from build123d import *

# Parameters (mm, degrees)
SKETCH_1_R               = 28.35
EXTRUDE_1_DEPTH          = 6
SKETCH_2_R               = 16
EXTRUDE_2_DEPTH          = 12
SKETCH_3_R               = 6.5
CUT_EXTRUDE_1_DEPTH      = 19
HOLE_WIZARD_M5_2_D       = 4.2
PATTERN_CIRCULAR_1_COUNT = 6
CUT_EXTRUDE_3_REACH      = 46.35
SKETCH_6_R               = 2.1


with BuildPart() as part:
    # Sketch 1 → Extrude 1 (new body)
    with BuildSketch(Plane.XY):
        Circle(SKETCH_1_R)
    extrude(amount=EXTRUDE_1_DEPTH)

    # Sketch 2 → Extrude 2 (add)
    with BuildSketch(Plane.XY.offset(6)):
        Circle(SKETCH_2_R)
    extrude(amount=EXTRUDE_2_DEPTH)

    # Sketch 3 → Cut-Extrude 1 (cut, through all)
    with BuildSketch(Plane.XY.offset(18)):
        Circle(SKETCH_3_R)
    extrude(amount=-CUT_EXTRUDE_1_DEPTH, mode=Mode.SUBTRACT)

    # Hole Wizard M5 _2 (through all)
    with Locations(Plane(origin=(0, 0, 0), x_dir=(-1, 0, 0), z_dir=(0, 0, -1))):
        with Locations((0, 23.75)):
            hole_wizard_m5_2 = Hole(HOLE_WIZARD_M5_2_D / 2)

    # Pattern Circular 1: Hole Wizard M5 _2 ×6 about axis
    pattern_circular_1_axis = Axis((0, 0, 0), (0, 0, 1))
    for i in range(1, PATTERN_CIRCULAR_1_COUNT):
        add(hole_wizard_m5_2.rotate(pattern_circular_1_axis, i * 360 / PATTERN_CIRCULAR_1_COUNT), mode=Mode.SUBTRACT)

    # Sketch 6 → Cut-Extrude 3 (cut, up to next)
    with BuildSketch(Plane(origin=(16, 0, 0), x_dir=(0, 0, -1), z_dir=(1, 0, 0)), mode=Mode.PRIVATE) as cut_extrude_3_sk1:
        with Locations((-11, 0)):
            Circle(SKETCH_6_R)
    cut_extrude_3_tool1 = extrude(cut_extrude_3_sk1.sketch, amount=-CUT_EXTRUDE_3_REACH, mode=Mode.PRIVATE) & part.part
    add(cut_extrude_3_tool1.solids().sort_by_distance((16, 0, 11))[0], mode=Mode.SUBTRACT)


solid = part.part
Could you check a few things on this model? Use its own coordinates, in mm. A direction names the side the tool comes from. Coordinates: 2 decimals unless noted, no trailing zeros. Write each loop counter-clockwise with the first axis right and the second up, starting at its lowest first coordinate (ties: lowest second). Pieces come first, ordered by that corner, then holes. Notation, with made-up numbers: M -11.75,-25 L 2.25,-25 A28 cw 2.25,5 Z; hole C 6.5,40 d6. An arc over 180 degrees is marked long. One line per question, with ' | ' between items.
1) Imagine slicing it at C-C, the plane z = 16. Write out the boundary of the cut face in (x, y), and give its area (3 significant figures).
Checks:
outline: C 0,0 d32; hole C 0,0 d13 | area: 672 mm²
2) Imagine slicing it at D-D, the plane x = 11. Write out the boundary of the cut face in (y, z), and give its area (3 significant figures).
Checks:
outline: M -26.13,0 L 26.13,0 L 26.13,6 L 11.62,6 L 11.62,18 L -11.62,18 L -11.62,6 L -26.13,6 Z; hole C 0,11 d4.2 | area: 579 mm²
3) I need wall thicknesses on probe 1 along Y at (x, z) = (0, 5.5); probe 2 along Z at (x, y) = (24.5, 13); probe 3 along X at (y, z) = (5.5, 10.75). Which ranges of each line are inside material? Lowest first, please. Write a range as [from, to].
Checks:
probe 1: [-28.35, -25.85], [-21.65, -6.5], [6.5, 21.65], [25.85, 28.35] | probe 2: [0, 6] | probe 3: [-15.02, -3.46], [3.46, 15.02]
4) Imagine slicing it at A-A, the plane x = 4. Write out the boundary of the cut face in (y, z), and give its area (3 significant figures).
Checks:
outline: M -28.07,0 L -5.12,0 L -5.12,18 L -15.49,18 L -15.49,6 L -28.07,6 Z; M 5.12,0 L 28.07,0 L 28.07,6 L 15.49,6 L 15.49,18 L 5.12,18 Z | area: 524 mm²
5) For pin 1 Ø10 at (y, z) = (15, 7.5) entering from -X; pin 2 Ø4 at (x, z) = (-11.5, 13.5) entering from -Y; pin 3 Ø10 at (x, z) = (18, 3) entering from +Y, each with a flat end and sliding along its axis, tell me the tip position at first contact or that it passes through.
Checks:
pin 1: x = -26.44 | pin 2: y = -12.87 | pin 3: y = 25.19
6) For faces 1 (the face through (11.14, 0.09, 13.1)), 2 (the face through (-5.158, -3.955, 9.126)), 3 (the face through (12, -12, 6)), which set-ups out of +Z, -Z, +X, -X, +Y, -Y let a thin tool reach every point of the face, with its end or its side?
Checks:
face 1: +X | face 2: +Z, -Z | face 3: +Z
7) If we mould it in two halves opening along Y, with no side actions, what happens to faces 4 (the face through (0, 7, 0)), 5 (the face through (-3.47, -15.62, 11.92)), 6 (the face through (18.47, -11.78, 3.04))? For each: released by +Y, released by -Y, zero draft, split by the parting line, or undercut.
Checks:
face 4: zero draft | face 5: split by the parting line | face 6: undercut
